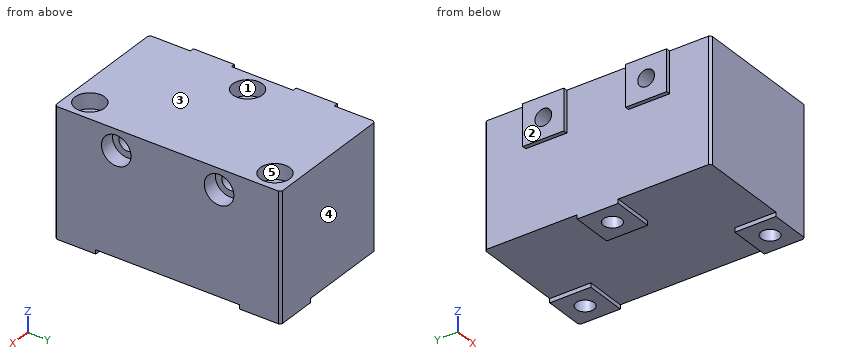
```python
from build123d import *

# Parameters (mm, degrees)
SKETCH1_W                                        = 81.534
SKETCH1_H                                        = 139.7
EXTRUDE1_DEPTH                                   = 76.2
SKETCH8_W                                        = 25.4
SKETCH8_H                                        = 25.4
EXTRUDE2_DEPTH                                   = 2.54
CBORE_FOR_3_8_SOCKET_HEAD_CAP_SCREW1_D           = 11.0998
CBORE_FOR_3_8_SOCKET_HEAD_CAP_SCREW1_CBORE_D     = 18.2626
CBORE_FOR_3_8_SOCKET_HEAD_CAP_SCREW1_CBORE_DEPTH = 9.525
SKETCH9_W                                        = 25.4
SKETCH9_H                                        = 25.4
EXTRUDE3_DEPTH                                   = 2.54
CBORE_FOR_3_8_SOCKET_HEAD_CAP_SCREW3_D           = 10.3124
CBORE_FOR_3_8_SOCKET_HEAD_CAP_SCREW3_CBORE_D     = 18.2626
CBORE_FOR_3_8_SOCKET_HEAD_CAP_SCREW3_CBORE_DEPTH = 9.525
CHAMFER1_SIZE                                    = 1.27


with BuildPart() as part:
    # Sketch1 → Extrude1 (new body)
    with BuildSketch(Plane.XY):
        with Locations((4.098167124, -35.572612746)):
            Rectangle(SKETCH1_W, SKETCH1_H)
    extrude(amount=EXTRUDE1_DEPTH)

    # Sketch8 → Extrude2 (add)
    with BuildSketch(Plane(origin=(0, 0, 0), x_dir=(-1, 0, 0), z_dir=(0, 0, -1))):
        with Locations((-32.165167124, -92.722612746)):
            Rectangle(SKETCH8_W, SKETCH8_H)
        with Locations((-32.165167124, 21.577387254)):
            Rectangle(SKETCH8_W, SKETCH8_H)
        with Locations((23.968832876, -35.572612746)):
            Rectangle(SKETCH8_W, SKETCH8_H)
    extrude(amount=EXTRUDE2_DEPTH)

    # CBORE for 3/8 Socket Head Cap Screw1 (through all)
    with Locations(Plane.XY.offset(76.2)):
        with Locations((-23.968832876, -35.572612746), (32.165167124, 21.577387254), (32.165167124, -92.722612746)):
            CounterBoreHole(CBORE_FOR_3_8_SOCKET_HEAD_CAP_SCREW1_D / 2, CBORE_FOR_3_8_SOCKET_HEAD_CAP_SCREW1_CBORE_D / 2, CBORE_FOR_3_8_SOCKET_HEAD_CAP_SCREW1_CBORE_DEPTH)

    # Sketch9 → Extrude3 (add)
    with BuildSketch(Plane.ZY.offset(36.668832876)):
        with Locations((63.5, -3.822612746)):
            Rectangle(SKETCH9_W, SKETCH9_H)
        with Locations((63.5, -67.322612746)):
            Rectangle(SKETCH9_W, SKETCH9_H)
    extrude(amount=EXTRUDE3_DEPTH)

    # CBORE for 3/8 Socket Head Cap Screw3 (through all)
    with Locations(Plane(origin=(44.865167124, 0, 0), x_dir=(0, 0, -1), z_dir=(1, 0, 0))):
        with Locations((-63.5, -3.822612746), (-63.5, -67.322612746)):
            CounterBoreHole(CBORE_FOR_3_8_SOCKET_HEAD_CAP_SCREW3_D / 2, CBORE_FOR_3_8_SOCKET_HEAD_CAP_SCREW3_CBORE_D / 2, CBORE_FOR_3_8_SOCKET_HEAD_CAP_SCREW3_CBORE_DEPTH)

    # Chamfer1
    chamfer1_edges = [part.edges().sort_by_distance(p)[0] for p in [
        (44.865167124, 34.277387254, 36.83),
        (-36.668832876, 34.277387254, 38.1),
        (44.865167124, -105.422612746, 36.83),
        (-36.668832876, -105.422612746, 38.1),
    ]]
    chamfer(chamfer1_edges, length=CHAMFER1_SIZE)


solid = part.part
```
Design review of the part built by this model. Coordinates are the model's own, in mm. Face numbers are marked on the shaded views. A direction names the side the tool comes from. Give positions to 0.01 mm unless a question says otherwise; leave off trailing zeros. Order: outer loops, then holes, each group sorted by start corner. A loop starts at its lowest first (then second) coordinate and runs counter-clockwise, first axis right, second up. Notation, with made-up numbers: (39, 72.25) -> (58, 72.25) arc R18 ccw to (58, 78.25) -> close; hole circle Ø4 at (56.25, -11). An arc over 180 degrees is marked (long way). Write each question's results on one line, items separated by ' | '. Start each with the question number.
Q1. Add section B-B on y = 25.5. Give the boundary of the cut face in (x, z) (3 decimals), and give its area (3 significant figures).
Q2. For pin 1 (2 mm diameter, centred on x = -37.5, y = -67, fed in from -Z); pin 2 (6 mm diameter, centred on y = 0, z = 37, fed in from -X); pin 3 (0.8 mm diameter, centred on y = -89, z = -1.5, fed in from -X), all flat-tipped, find the tip position at first contact; note any pin that passes through.
Q3. Add section C-C on z = 44. Give the boundary of the cut face in (x, y), and give its area (3 significant figures).
Q4. Mouldability with a two-part tool opening along Y and no side actions: class the marked faces 3, 4 and 5 as +Y half, -Y half, draft (parallel to the pull), parting line (faces both ways), or undercut.
Q5. Add section D-D on x = 5. Give the boundary of the cut face in (y, z).
Q6. Add section A-A on x = -22. Give the boundary of the cut face in (y, z) (3 decimals), and give its area (3 significant figures).
Q7. Wall thickness on L1, parallel to Y at x = 41, z = 63; L2, parallel to Y at x = 38.75, z = 63.5; L3, parallel to X at y = -92, z = 72: over which ranges is each line inside the solid? List them lowest first. Write a range as from..to.
Q8. Machinability: for the marked faces 1 and 2, which of the approach directions +Z, -Z, +X, -X, +Y, -Y give a long, thin tool a straight path to every point of the face, cutting with its end or side? Answer none if there is none.
Found:
1) outline: (-36.669, 0) -> (19.465, 0) -> (19.465, -2.54) -> (28.239, -2.54) -> (28.239, 66.675) -> (23.919, 66.675) -> (23.919, 76.2) -> (-36.669, 76.2) -> close; (36.091, -2.54) -> (44.865, -2.54) -> (44.865, 76.2) -> (40.411, 76.2) -> (40.411, 66.675) -> (36.091, 66.675) -> close | area: 5,580 mm2
2) pin 1: stops at z = 0 | pin 2: stops at x = -36.67 | pin 3: stops at x = 19.47
3) outline: (-36.67, -104.15) -> (-35.4, -105.42) -> (43.6, -105.42) -> (44.87, -104.15) -> (44.87, 33.01) -> (43.6, 34.28) -> (-35.4, 34.28) -> (-36.67, 33.01) -> close; hole circle Ø11.1 at (-23.97, -35.57); hole circle Ø11.1 at (32.17, -92.72); hole circle Ø11.1 at (32.17, 21.58) | area: 11,100 mm2
4) face 3: draft | face 4: +Y half | face 5: undercut
5) outline: (-105.42, 0) -> (34.28, 0) -> (34.28, 76.2) -> (-105.42, 76.2) -> close; hole circle Ø10.31 at (-67.32, 63.5); hole circle Ø10.31 at (-3.82, 63.5)
6) outline: (-105.423, 0) -> (-48.273, 0) -> (-48.273, -2.54) -> (-40.762, -2.54) -> (-40.762, 66.675) -> (-44.489, 66.675) -> (-44.489, 76.2) -> (-105.423, 76.2) -> close; (-30.384, -2.54) -> (-22.873, -2.54) -> (-22.873, 0) -> (34.277, 0) -> (34.277, 76.2) -> (-26.656, 76.2) -> (-26.656, 66.675) -> (-30.384, 66.675) -> close; hole circle Ø10.312 at (-67.323, 63.5); hole circle Ø10.312 at (-3.823, 63.5) | area: 9,650 mm2
7) L1: y = -105.42..-76.44, -58.21..-12.94, 5.29..34.28 | L2: y = -105.42..-76.45, -58.19..-12.95, 5.31..34.28 | L3: x = -36.67..23.06, 41.27..44.87
8) face 1: +Z | face 2: +Z, -Z, -X, +Y, -Y
